Autodesk Inventor part; units mm, degrees
ref_plane "YZ Plane" through (0, 0, 0) normal (1, 0, 0) x (0, 1, 0)
ref_plane "XZ Plane" through (0, 0, 0) normal (0, 1, 0) x (-1, 0, 0)
ref_plane "XY Plane" through (0, 0, 0) normal (0, 0, 1) x (1, 0, 0)
sketch "Sketch1" plane through (0, 0, 0) normal (0, 0, 1) x (1, 0, 0)
  circle A0 centre (0, 0) radius 3
  dimension "d0" = 6
extrude "Extrusion1" add sketch "Sketch1" along normal blind 5
sketch "Sketch2" plane through (0, 0, 5) normal (0, 0, 1) x (1, 0, 0)
  circle A0 centre (0, 0) radius 3
  line L0 (0, 0) -> (-12, 0)
  circle A1 centre (-12, 0) radius 0.5
  circle A2 centre (-12, 0) radius 2.25
  line L1 (-0.1875, -2.9941) -> (-12.1406, -2.2456)
  line L2 (-12.1406, 2.2456) -> (-0.1875, 2.9941)
  circle A3 centre (0, 0) radius 3
  dimension "d3" = 12
  dimension "d4" = 1
  dimension "d5" = 4.5
extrude "Extrusion2" add sketch "Sketch2" against normal blind 1.5 contours A0 L0 A2 L2 | L1 A2 L0 A0 | A2
properties part number "ServoArm"
Read the model definition and answer for the solid it produces. Units are mm, in the model's axes. Coordinates: 2 decimals unless noted, no trailing zeros. Order: outer loops, then holes, each group sorted by start corner. A loop starts at its lowest first (then second) coordinate and runs counter-clockwise, first axis right, second up. Notation, with made-up numbers: (16, -2.5) - (32, -2.5) arc R23 cw to (32, 23.5) - close; hole circle Ø3 at (-35.75, -28). An arc over 180 degrees is marked (long way). Use one line per item in the form item = value.
(1) Given pin 1 Ø3 at (x, y) = (-4.5, -2) entering from -Z; pin 2 Ø1 at (y, z) = (1, 4) entering from -X; pin 3 Ø1 at (y, z) = (-2, 2.5) entering from +X, each flat-ended and moving along its own axis, determine where each tip first touches the part or whether it passes through.
Computed values:
pin_1 = 3.5
pin_2 = -14.19
pin_3 = 2.6
(2) Section B-B, the plane y = 0.2 is taken. Give the vertices of the cut face in (x, z).
Computed values:
outline = (-14.24, 3.5) - (-12.46, 3.5) - (-12.46, 5) - (-14.24, 5) - close; (-11.54, 3.5) - (-2.99, 3.5) - (-2.99, 0) - (2.99, 0) - (2.99, 5) - (-11.54, 5) - close
(3) Straight lines are drawn through the part: L1, parallel to Z at x = -3.75, y = -0.9; L2, parallel to X at y = 0, z = 2.4; L3, parallel to Y at x = -12, z = 3.85. For each, find the intervals that lie inside material, in ascending order.
Computed values:
L1 = 3.5 to 5
L2 = -3 to 3
L3 = -2.25 to -0.5, 0.5 to 2.25
(4) For a pull along X with two mould halves and no side action, classify faces 1 (the face through (2.77, 1.15, 1.91)), 2 (the face through (-6, 0, 5)), 3 (the face through (-6.08, -2.625, 4.26)), 4 (the face through (-12.5, 0, 4.3)) as pulls with the +X half, pulls with the -X half, needs draft (parallel to the pull), parting line crosses it, or undercut.
Computed values:
face_1 = parting line crosses it
face_2 = needs draft
face_3 = pulls with the -X half
face_4 = undercut
(5) Section C-C, the plane y = -2.6 is taken. Give the vertices of the cut face in (x, z), then the cut area to 3 significant figures.
Computed values:
outline = (-6.48, 3.5) - (-1.5, 3.5) - (-1.5, 0) - (1.5, 0) - (1.5, 5) - (-6.48, 5) - close
area = 22.4 mm²
(6) Section D-D, the plane z = 2.05 is taken. Give the vertices of the cut face in (x, y).
Computed values:
outline = circle Ø6 at (0, 0)
